from build123d import *

# Parameters (mm, degrees)
SKETCH1_R           = 1.25
SKETCH1_R_2         = 1.7
BOSS_EXTRUDE1_DEPTH = 3.175


with BuildPart() as part:
    # Sketch1 → Boss-Extrude1 (new body)
    with BuildSketch(Plane(origin=(0, 0, 0), x_dir=(1, 0, 0), z_dir=(0, 1, 0))):
        with BuildLine():
            Line((4.709206507, -2.660218653), (34.68016435, -2.660218653))
            ThreePointArc((34.68016435, -2.660218653), (36.801406663, -1.781571318), (37.680053998, 0.339670996))
            Line((37.680053998, 0.339670996), (37.680053998, 18.345692352))
            ThreePointArc((37.680053998, 18.345692352), (36.802919812, 20.463281602), (34.685330562, 21.340415789))
            add(Edge.make_bspline(
                [(34.685330562, 21.340415789), (13.555998876, 21.34041579), (5.457536405, 21.34041579)],
                knots=[8, 8, 8, 9, 9, 9], degree=2))
            ThreePointArc((5.457536405, 21.34041579), (3.903764208, 22.107666003), (2.349992011, 21.34041579))
            Line((2.349992011, 21.34041579), (-10.092264133, 20.808084054))
            ThreePointArc((-10.092264133, 20.808084054), (-12.117989286, 19.884860301), (-12.930141677, 17.812105374))
            Line((-12.930141677, 17.812105374), (-12.916142632, 0.575581301))
            ThreePointArc((-12.916142632, 0.575581301), (-12.012905856, -1.307536184), (-10.092264134, -2.127965046))
            Line((-10.092264134, -2.127965046), (2.059487443, -2.660218653))
            ThreePointArc((2.059487443, -2.660218653), (3.384346975, -3.471607461), (4.709206507, -2.660218653))
        make_face()
        with Locations(Location((-10.13526538, 17.840261618, 0), (0, 0, 270))):
            Circle(SKETCH1_R, mode=Mode.SUBTRACT)
        with Locations(Location((-10.13526538, 0.839730428, 0), (0, 0, 270))):
            Circle(SKETCH1_R, mode=Mode.SUBTRACT)
        with Locations(Location((19.41222808, 0.839632764, 0), (0, 0, 270))):
            Circle(SKETCH1_R, mode=Mode.SUBTRACT)
        with Locations(Location((19.412228081, 17.840168837, 0), (0, 0, 270))):
            Circle(SKETCH1_R, mode=Mode.SUBTRACT)
        with Locations(Location((34.685233075, 0.289707036, 0), (0, 0, 270))):
            Circle(SKETCH1_R_2, mode=Mode.SUBTRACT)
        with Locations(Location((34.685264759, 18.390319188, 0), (0, 0, 270))):
            Circle(SKETCH1_R_2, mode=Mode.SUBTRACT)
        Polygon((12.275095957, 3.139860204), (12.225070816, 3.139860204), (12.225070816, 0.139779677), (-5.243817542, 0.139779677), (-5.243817542, 3.139860204), (-7.938965263, 3.139860204), (-7.938965263, 15.540268571), (-2.448882753, 15.540268571), (-2.448882753, 18.540349097), (9.530118068, 18.540349097), (9.530118068, 15.540268571), (15.020200579, 15.540268571), (15.020200579, 3.139860204), align=None, mode=Mode.SUBTRACT)
    extrude(amount=BOSS_EXTRUDE1_DEPTH)


solid = part.part
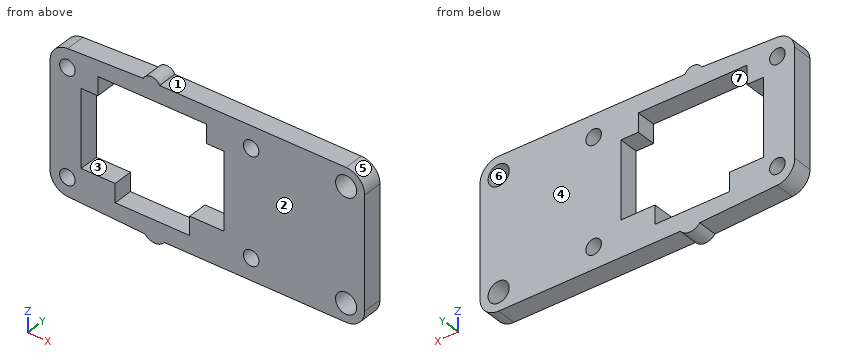
Could you check a few things on this model? Use its own coordinates, in mm. Face numbers are marked on the shaded views. A direction names the side the tool comes from. Round coordinates to 2 decimals unless told otherwise and drop trailing zeros. Write each loop counter-clockwise with the first axis right and the second up, starting at its lowest first coordinate (ties: lowest second). Pieces come first, ordered by that corner, then holes. Notation, with made-up numbers: (67.25, 0.5) - (84.25, 0.5) arc R18 ccw to (84.25, 14.5) - close; hole circle Ø2 at (45, -37.75). An arc over 180 degrees is marked (long way). Put each result on its own line as item: value. Start each with the question number.
(1) I need wall thicknesses on probe 1 along X at (y, z) = (0.3, -4.5); probe 2 along X at (y, z) = (2.3, -1.5); probe 3 along Z at (x, y) = (27.5, 2.5). Which ranges of each line are inside material? Lowest first, please.
(2) Thinking about a two-plate mould opening in X: for the marked faces 4, 5, 6 and 7, which applies, released by +X, released by -X, zero draft, split by the parting line, or undercut?
(3) For the marked faces 1, 2 and 3, which set-ups out of +Z, -Z, +X, -X, +Y, -Y let a thin tool reach every point of the face, with its end or its side?
(4) I want a section at C-C, the plane y = 0.9. Give the number of separate pieces and of enclosed holes in the cut face, plus the area to 3 significant figures.
(5) I want a section at A-A, the plane x = 1. Please give me the cut outline in (y, z) (3 decimals), plus the area to 3 significant figures.
(6) Will these pins go through, and if not, where does the flat tip stop? pin 1 (1.5 mm diameter, centred on y = 1.5, z = -19.5, fed in from +X); pin 2 (1.4 mm diameter, centred on x = 13.5, y = 1, fed in from -Z); pin 3 (1 mm diameter, centred on y = 2, z = -9, fed in from -X).
(7) I want a section at B-B, the plane z = -7. Please give me the cut outline in (x, y) (3 decimals), plus the area to 3 significant figures.
Here are the results:
1. probe 1: x = -12.92 to -7.94, 15.02 to 37.68
1. probe 2: x = -12.92 to -11.2, -9.07 to -5.24, 12.23 to 18.35, 20.47 to 33.49, 35.88 to 37.68
1. probe 3: z = -21.34 to 2.66
2. face 4: zero draft
2. face 5: released by +X
2. face 6: undercut
2. face 7: undercut
3. face 1: +Z, +X, +Y, -Y
3. face 2: +Z, -Z, +X, -X, -Y
3. face 3: +Y, -Y
4. separate pieces: 1
4. enclosed holes: 7
4. area: 790 mm^2
5. outline: (0, -21.283) - (3.175, -21.283) - (3.175, -18.54) - (0, -18.54) - close; (0, -0.14) - (3.175, -0.14) - (3.175, 2.614) - (0, 2.614) - close
5. area: 17.4 mm^2
6. pin 1: stops at x = 37.65
6. pin 2: stops at z = -21.34
6. pin 3: stops at x = -12.92
7. outline: (-12.921, 0) - (-7.939, 0) - (-7.939, 3.175) - (-12.921, 3.175) - close; (15.02, 0) - (37.68, 0) - (37.68, 3.175) - (15.02, 3.175) - close
7. area: 87.8 mm^2
